The listing builds one solid part. Answer for the finished solid, in the listing's coordinates (mm). A direction names the side the tool comes from. Coordinates: 2 decimals unless noted, no trailing zeros. Order: outer loops, then holes, each group sorted by start corner. A loop starts at its lowest first (then second) coordinate and runs counter-clockwise, first axis right, second up.
Autodesk Inventor part; units mm, degrees
ref_plane "YZ Plane" through (0, 0, 0) normal (1, 0, 0) x (0, 1, 0)
ref_plane "XZ Plane" through (0, 0, 0) normal (0, 1, 0) x (-1, 0, 0)
ref_plane "XY Plane" through (0, 0, 0) normal (0, 0, 1) x (1, 0, 0)
sketch "スケッチ1" plane through (0, 0, 0) normal (1, 0, 0) x (0, 1, 0)
  line L0 (-19.75, 0) -> (19.75, 0)
  line L1 (0, 0) -> (0, 3.4641) construction
  line L2 (-19.4821, 3.4641) -> (-19.75, 3)
  line L3 (-19.75, 3) -> (-19.75, 0)
  line L4 (-19.4821, 3.4641) -> (19.4821, 3.4641)
  line L5 (19.4821, 3.4641) -> (19.75, 3)
  line L6 (19.75, 3) -> (19.75, 0)
  dimension "d1" = 3
  dimension "d2" = 3.4641
  dimension "d3" = 30
  dimension "d4" = 39.5
revolve "回転1" add sketch "スケッチ1" angle 360 about axis through (0, -19.75, 0) along (0, 1, 0)
sketch "スケッチ2" plane through (0, 19.75, 0) normal (0, 1, 0) x (1, 0, 0)
  circle A0 centre (0, 0) radius 3.4641
  line L0 (0, -3.4641) -> (-3, -1.7321)
  line L1 (-3, -1.7321) -> (-3, 1.7321)
  line L2 (-3, 1.7321) -> (0, 3.4641)
  line L3 (0, 3.4641) -> (3, 1.7321)
  line L4 (3, 1.7321) -> (3, -1.7321)
  line L5 (3, -1.7321) -> (0, -3.4641)
  point P0 (0, 0)
  point P1 (0, 0)
  point P2 (3, -1.7321)
  point P3 (3, -1.7321)
  point P4 (3, 1.7321)
  point P5 (3, 1.7321)
  point P6 (0, 3.4641)
  point P7 (0, 3.4641)
  point P8 (-3, 1.7321)
  point P9 (-3, 1.7321)
  point P10 (-3, -1.7321)
  point P11 (-3, -1.7321)
  point P12 (0, 0)
extrude "押し出し1" cut sketch "スケッチ2" against normal through all contours A0 L4 | L3 A0 | A0 L5 | L2 A0 | A0 L0 | L1 A0
hole "穴1" at (0, 19.75, 0) direction (0, -1, 0) diameter 3.242 depth 11.8 tip angle 118 countersink diameter 4 countersink angle 90
mirror "ミラー1" about plane through (0, 0, 0) normal (0, 1, 0) of "穴1"
equation "\"d2\" = 1.1547 * d1"
properties part number "SLSBF6-39.5-M4-N4" material "ステンレス鋼 AISI 304"
1) A cutting plane is placed at A-A, the plane y = 17. Write down the section's boundary in (x, z).
2) The mould has two halves that part along Z. Classify faces 4 (the conical face through (-0.069, -19.674, 3.131)), 5 (the conical face through (0.069, -19.674, -3.131)), 6 (the conical face through (-0.275, 7.145, -0.061)): released by +Z, released by -Z, zero draft, split by the parting line, or undercut.
3) Each of these flat-tipped pins is pushed along its axis until it touches: P1, Ø3, axis at x = 0, z = 0, coming from the -Y side; P2, Ø2.5, axis at x = 0, z = 0, coming from the -Y side. Where does it stop, or does it pass through?
4) Straight lines are drawn through the part: probe 1 along X at (y, z) = (-16.25, 0); probe 2 along Z at (x, y) = (2.55, -1); probe 3 along Z at (x, y) = (-0.4, 7.5). For each, find the intervals that lie inside material, in ascending order.
5) For faces 1 (the flat face through (1.5, 0.3, -2.6)), 2 (the cylindrical face through (1.438, 13.581, 0.748)), 3 (the cylindrical face through (-1.438, -13.581, 0.748)), determine the directions among +Z, -Z, +X, -X, +Y, -Y from which every point of the face is accessible in a straight line to the end or side of a thin tool.
Working result:
1. outline: (-3, -1.73) - (0, -3.46) - (3, -1.73) - (3, 1.73) - (0, 3.46) - (-3, 1.73) - close; hole circle Ø3.24 at (0, 0)
2. face 4: released by +Z
2. face 5: released by -Z
2. face 6: undercut
3. P1: stops at y = -7.88
3. P2: stops at y = -7.73
4. probe 1: x = -3 to -1.62, 1.62 to 3
4. probe 2: z = -1.99 to 1.99
4. probe 3: z = -3.23 to -0.77, 0.77 to 3.23
5. face 1: -Z, +X, +Y, -Y
5. face 2: +Y
5. face 3: -Y
